The model under review builds one solid part; all positions refer to its coordinate system, in mm. Give positions to 0.01 mm unless a question says otherwise; leave off trailing zeros. Order: outer loops, then holes, each group sorted by start corner. A loop starts at its lowest first (then second) coordinate and runs counter-clockwise, first axis right, second up. Notation, with made-up numbers: (51.5, 49) - (86.5, 49) arc R3 ccw to (86.5, 54) - close; hole circle Ø7 at (61.5, 59.5). An arc over 180 degrees is marked (long way). Use CSV: the item, a comma, the result in double quotes. Start each with the question number.
1. To check wall thickness, follow line 1 (Y direction, x = -151.5, z = 139.45); line 2 (Y direction, x = -151.5, z = 134); line 3 (Z direction, x = -154.25, y = -35). State the ranges of each line that lie inside material, in increasing order. Write a range as [from, to].
2. For pin 1 (2.5 mm diameter, centred on x = -155, y = 17.5, fed in from -Z); pin 2 (4 mm diameter, centred on x = -151.5, y = 0, fed in from -Z); pin 3 (1.8 mm diameter, centred on y = -20, z = 121, fed in from -X); pin 4 (3 mm diameter, centred on x = -151.5, y = 0, fed in from +Z), all flat-tipped, find the tip position at first contact; note any pin that passes through.
3. Take a section at C-C, the plane y = -9. State the section outline as (x, z) points, then the cut area to 3 significant figures.
4. Take a section at A-A, the plane y = 0. State the section outline as (x, z) points, then the cut area to 3 significant figures.
5. Take a section at B-B, the plane x = -151.5. State the section outline as (y, z) points.
```python
from build123d import *

# Parameters (mm, degrees)
MAIN_PROFILE_SKETCH_W     = 8
MAIN_PROFILE_SKETCH_H     = 86
MAIN_PROFILE_SKETCH_R     = 3
MAIN_EXTRUSION_DEPTH      = 2
DETAIL_PROFILE_2_SKETCH_W = 8
DETAIL_PROFILE_2_SKETCH_H = 86
DETAIL_PROFILE_2_SKETCH_R = 1.7
DETAIL_EXTRUSION_2_DEPTH  = 15.8
DETAIL_PROFILE_3_SKETCH_W = 5.9
DETAIL_PROFILE_3_SKETCH_H = 86
DETAIL_PROFILE_3_SKETCH_R = 1.7
DETAIL_EXTRUSION_3_DEPTH  = 2.2


with BuildPart() as part:
    # Main Profile Sketch → Main Extrusion (new body)
    with BuildSketch(Plane.XY.offset(140)):
        with Locations((-151.5, 0)):
            Rectangle(MAIN_PROFILE_SKETCH_W, MAIN_PROFILE_SKETCH_H)
        with Locations((-151.5, 0)):
            Circle(MAIN_PROFILE_SKETCH_R, mode=Mode.SUBTRACT)
    extrude(amount=-MAIN_EXTRUSION_DEPTH)

    # Detail Profile 2 Sketch → Detail Extrusion 2 (add)
    with BuildSketch(Plane.XY.offset(138)):
        with Locations((-151.5, 0)):
            Rectangle(DETAIL_PROFILE_2_SKETCH_W, DETAIL_PROFILE_2_SKETCH_H)
        with Locations((-151.5, 0)):
            Circle(DETAIL_PROFILE_2_SKETCH_R, mode=Mode.SUBTRACT)
    extrude(amount=-DETAIL_EXTRUSION_2_DEPTH)

    # Detail Profile 3 Sketch → Detail Extrusion 3 (add)
    with BuildSketch(Plane.XY.offset(122.2)):
        with Locations((-150.45, 0)):
            Rectangle(DETAIL_PROFILE_3_SKETCH_W, DETAIL_PROFILE_3_SKETCH_H)
        with Locations((-151.5, 0)):
            Circle(DETAIL_PROFILE_3_SKETCH_R, mode=Mode.SUBTRACT)
    extrude(amount=-DETAIL_EXTRUSION_3_DEPTH)


solid = part.part
```
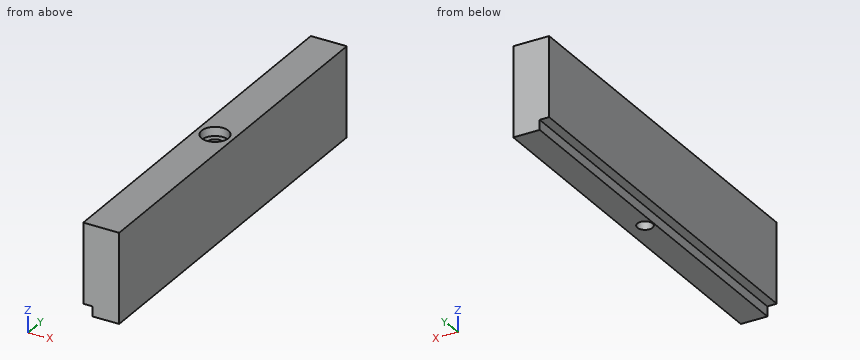
Determined:
1,line 1,"y = [-43, -3], [3, 43]"
1,line 2,"y = [-43, -1.7], [1.7, 43]"
1,line 3,"z = [122.2, 140]"
2,pin 1,"stops at z = 122.2"
2,pin 2,"stops at z = 120"
2,pin 3,"stops at x = -153.4"
2,pin 4,"passes through"
3,outline,"(-155.5, 122.2) - (-153.4, 122.2) - (-153.4, 120) - (-147.5, 120) - (-147.5, 140) - (-155.5, 140) - close"
3,area,"155 mm²"
4,outline,"(-155.5, 122.2) - (-153.4, 122.2) - (-153.4, 120) - (-153.2, 120) - (-153.2, 138) - (-154.5, 138) - (-154.5, 140) - (-155.5, 140) - close; (-149.8, 120) - (-147.5, 120) - (-147.5, 140) - (-148.5, 140) - (-148.5, 138) - (-149.8, 138) - close"
4,area,"82.2 mm²"
5,outline,"(-43, 120) - (-1.7, 120) - (-1.7, 138) - (-3, 138) - (-3, 140) - (-43, 140) - close; (1.7, 120) - (43, 120) - (43, 140) - (3, 140) - (3, 138) - (1.7, 138) - close"
